from build123d import *

# Parameters (mm, degrees)
SKETCH_W    = 156
SKETCH_H    = 156
PAD_DEPTH   = 50
THICKNESS_T = -2


with BuildPart() as part:
    # Sketch → Pad (new body)
    with BuildSketch(Plane.XY):
        Rectangle(SKETCH_W, SKETCH_H)
    extrude(amount=PAD_DEPTH)

    # Thickness
    thickness_openings = [part.faces().sort_by_distance(p)[0] for p in [
        (0, 0, 50),
    ]]
    offset(amount=THICKNESS_T, openings=thickness_openings)


solid = part.part
The model under review builds one solid part; all positions refer to its coordinate system, in mm. A direction names the side the tool comes from. Give positions to 0.01 mm unless a question says otherwise; leave off trailing zeros. Loops run counter-clockwise (first coordinate to the right, second up) from the corner with the lowest first, then second, coordinate; pieces in that order, holes last. Notation, with made-up numbers: (-15, 14.5) -> (19, 14.5) arc R32 cw to (19, 49.5) -> close; hole circle Ø2 at (10, 41). An arc over 180 degrees is marked (long way). Put each result on its own line as item: value. Start each with the question number.
1. Wall thickness on probe 1 along X at (y, z) = (-43, 14); probe 2 along Z at (x, y) = (-1.5, 51): over which ranges is each line inside the solid? List them lowest first.
2. Mouldability with a two-part tool opening along Y and no side actions: class faces 3 (the face through (-1, 1, 0)), 4 (the face through (-1, -78, 25)), 5 (the face through (-1, 1, 2)) as released by +Y, released by -Y, zero draft, split by the parting line, or undercut.
3. Clearance check with a flat-ended pin moving along its axis: P1, Ø6, axis at x = -41.5, y = -18.5, coming from the +Z side. State where the tip first meets the part, or that it passes through.
4. We need section B-B on y = 21. State the section outline as (x, z) points, then the cut area to 3 significant figures.
5. For faces 1 (the face through (78, -1, 25)), 2 (the face through (-76, -1, 26)), list the 3-axis set-ups (+Z, -Z, +X, -X, +Y, -Y) from which the entire face can be reached by the end or side of a thin tool; tool diameter is ignored.
6. We need section A-A on z = 20.5. State the section outline as (x, y) points, then the cut area to 3 significant figures.
Determined:
1. probe 1: -78 to -76, 76 to 78
1. probe 2: 0 to 2
2. face 3: zero draft
2. face 4: released by -Y
2. face 5: undercut
3. P1: z = 2
4. outline: (-78, 0) -> (78, 0) -> (78, 50) -> (76, 50) -> (76, 2) -> (-76, 2) -> (-76, 50) -> (-78, 50) -> close
4. area: 504 mm^2
5. face 1: +Z, -Z, +X, +Y, -Y
5. face 2: +Z
6. outline: (-78, -78) -> (78, -78) -> (78, 78) -> (-78, 78) -> close; hole (-76, -76) -> (76, -76) -> (76, 76) -> (-76, 76) -> close
6. area: 1,230 mm^2
